```python
from build123d import *

# Parameters (mm, degrees)
SKETCH_1_W            = 101.6
SKETCH_1_H            = 101.6
EXTRUDE_1_DEPTH       = 2.9718
CUT_EXTRUDE_1_DEPTH   = 144.714827333
MIRROR_2_COPY_1_DEPTH = 144.714827333
CUT_EXTRUDE_3_DEPTH   = 144.714827333
SKETCH_2_W            = 101.6
SKETCH_2_H            = 2.9718
CUT_EXTRUDE_4_DEPTH   = 2.9718


with BuildPart() as part:
    # 草图1 → 凸台-拉伸1 (new body)
    with BuildSketch(Plane(origin=(0, 0, 0), x_dir=(1, 0, 0), z_dir=(0, 1, 0))):
        with Locations((50.8, 50.8)):
            Rectangle(SKETCH_1_W, SKETCH_1_H)
    extrude(amount=EXTRUDE_1_DEPTH)

    # 草图1<3> → 切除-拉伸1 (cut, through all)
    with BuildSketch(Plane(origin=(0, 0, 0), x_dir=(1, 0, 0), z_dir=(0, 1, 0))):
        Polygon((37.676666667, 98.6282), (37.676666667, 101.6), (30.056666667, 101.6), (30.056666667, 98.6282), (31.866666667, 98.6282), (31.866666667, 93.6282), (29.866666667, 93.6282), (29.866666667, 90.6282), (31.866666667, 90.6282), (31.866666667, 86.6282), (35.866666667, 86.6282), (35.866666667, 90.6282), (37.866666667, 90.6282), (37.866666667, 93.6282), (35.866666667, 93.6282), (35.866666667, 98.6282), align=None)
    cut_extrude_1 = extrude(amount=CUT_EXTRUDE_1_DEPTH, mode=Mode.SUBTRACT)

    # 镜向1: 切除-拉伸1 across plane
    add(cut_extrude_1.mirror(Plane(origin=(0, 0, -50.8), x_dir=(1, 0, 0), z_dir=(0, 0, -1))), mode=Mode.SUBTRACT)

    # 镜向2: 切除-拉伸1 across plane
    add(cut_extrude_1.mirror(Plane(origin=(50.8, 0, 0), x_dir=(0, 0, 1), z_dir=(1, 0, 0))), mode=Mode.SUBTRACT)

    # 镜向2 copy 1 sketch → 镜向2 copy 1 (cut, through all)
    with BuildSketch(Plane(origin=(101.6, 0, -101.6), x_dir=(-1, 0, 0), z_dir=(0, 1, 0))):
        Polygon((37.676666667, 98.6282), (37.676666667, 101.6), (30.056666667, 101.6), (30.056666667, 98.6282), (31.866666667, 98.6282), (31.866666667, 93.6282), (29.866666667, 93.6282), (29.866666667, 90.6282), (31.866666667, 90.6282), (31.866666667, 86.6282), (35.866666667, 86.6282), (35.866666667, 90.6282), (37.866666667, 90.6282), (37.866666667, 93.6282), (35.866666667, 93.6282), (35.866666667, 98.6282), align=None)
    extrude(amount=MIRROR_2_COPY_1_DEPTH, mode=Mode.SUBTRACT)

    # 草图1<4> → 切除-拉伸3 (cut, through all)
    with BuildSketch(Plane(origin=(0, 0, 0), x_dir=(1, 0, 0), z_dir=(0, 1, 0))):
        Polygon((0, 71.543333333), (0, 63.923333333), (2.9718, 63.923333333), (2.9718, 65.733333333), (7.9718, 65.733333333), (7.9718, 63.733333333), (10.9718, 63.733333333), (10.9718, 65.733333333), (14.9718, 65.733333333), (14.9718, 69.733333333), (10.9718, 69.733333333), (10.9718, 71.733333333), (7.9718, 71.733333333), (7.9718, 69.733333333), (2.9718, 69.733333333), (2.9718, 71.543333333), align=None)
    cut_extrude_3 = extrude(amount=CUT_EXTRUDE_3_DEPTH, mode=Mode.SUBTRACT)

    # 镜向3: 切除-拉伸3 across plane
    add(cut_extrude_3.mirror(Plane(origin=(0, 0, -50.8), x_dir=(1, 0, 0), z_dir=(0, 0, -1))), mode=Mode.SUBTRACT)

    # 草图2 → 切除-拉伸4 (cut)
    with BuildSketch(Plane(origin=(101.6, 0, 0), x_dir=(0, 0, -1), z_dir=(1, 0, 0))):
        with Locations((50.8, 1.4859)):
            Rectangle(SKETCH_2_W, SKETCH_2_H)
    extrude(amount=-CUT_EXTRUDE_4_DEPTH, mode=Mode.SUBTRACT)


solid = part.part
```
Geometry check sheet. Reference: the model listing, model coordinates, mm. A direction names the side the tool comes from. Round coordinates to 2 decimals unless told otherwise and drop trailing zeros. Loops run counter-clockwise (first coordinate to the right, second up) from the corner with the lowest first, then second, coordinate; pieces in that order, holes last. Notation, with made-up numbers: M 52.25,40 L 82.25,40 A30 ccw 82.25,66 Z; hole C 82.25,23 d5. An arc over 180 degrees is marked long. Return JSON: item names as keys, results as strings. Group by question number.
(1) Section check A-A, the plane x = 33.5. Enter the section's corners in (y, z), and give its area (3 significant figures).
(2) Set-up check for faces 4 (the face through (15, 1, 0)), 5 (the face through (34, 1, -14.972)), 6 (the face through (35.867, 1, -89)), 7 (the face through (9, 1, -37.867)), 8 (the face through (2, 1, -71.543)): record each of +Z, -Z, +X, -X, +Y, -Y from which the full face is reachable in a straight line by a thin tool's end or side.
(3) Mould release check, pull along Z, two halves, no side actions. Record for faces 1 (the face through (37.677, 1, -2)), 2 (the face through (71.733, 1, -9)), 3 (the face through (85, 1, 0)): pulls with the +Z half, pulls with the -Z half, needs draft (parallel to the pull), parting line crosses it, or undercut.
(4) Go/stop test with a flat-tipped pin: pin 1 (0.9 mm diameter, centred on x = 71, y = 1.5, fed in from -Z). Record where the tip stops, or that it passes through.
(5) Scan lines: line 1 along X through (y, z) = (0.8, -13); line 2 along Z through (x, y) = (14, 0.7); line 3 along Z through (x, y) = (10, 2.65). Record each from-to range of solid material in increasing order. Write a range as [from, to].
Data:
{
 "1": {"outline": "M 0,-86.63 L 2.97,-86.63 L 2.97,-14.97 L 0,-14.97 Z", "area": "213 mm²"},
 "2": {"face 4": "+Z, +X, -X, +Y, -Y", "face 5": "+Z, +Y, -Y", "face 6": "-Z, +Y, -Y", "face 7": "+Y, -Y", "face 8": "-X, +Y, -Y"},
 "3": {"face 1": "needs draft", "face 2": "undercut", "face 3": "pulls with the +Z half"},
 "4": {"pin 1": "z = -98.63"},
 "5": {"line 1": "[0, 31.87], [35.87, 65.73], [69.73, 98.63]", "line 2": "[-101.6, -69.73], [-65.73, -35.87], [-31.87, 0]", "line 3": "[-101.6, -71.73], [-63.73, -37.87], [-29.87, 0]"}
}
